```python
from build123d import *

# Parameters (mm, degrees)
F0_R     = 1.6
F1_DEPTH = 3


with BuildPart() as f1:
    # F0 (on Top) → F1 (new body)
    with BuildSketch(Plane.XY):
        with BuildLine():
            ThreePointArc((19.037183, -8.147739), (21.912225, -8.930193), (24.043754, -6.848203))
            ThreePointArc((24.043754, -6.848203), (24.759784, -3.457322), (25, 0))
            ThreePointArc((25, 0), (-19.952507, 15.063116), (6.848203, -24.043754))
            ThreePointArc((6.848203, -24.043754), (8.930193, -21.912225), (8.147739, -19.037183))
            Line((8.147739, -19.037183), (-5.444722, -5.444722))
            ThreePointArc((-5.444722, -5.444722), (-5.444722, 5.444722), (5.444722, 5.444722))
            Line((5.444722, 5.444722), (19.037183, -8.147739))
        make_face()
        with Locations((0, -20)):
            Circle(F0_R, mode=Mode.SUBTRACT)
        with Locations((-20, 0)):
            Circle(F0_R, mode=Mode.SUBTRACT)
        with Locations((20, 0)):
            Circle(F0_R, mode=Mode.SUBTRACT)
        with Locations((0, 20)):
            Circle(F0_R, mode=Mode.SUBTRACT)
        with BuildLine():
            ThreePointArc((6.848203, -24.043754), (17.67767, -17.67767), (24.043754, -6.848203))
            ThreePointArc((24.043754, -6.848203), (21.912225, -8.930193), (19.037183, -8.147739))
            Line((19.037183, -8.147739), (5.444722, 5.444722))
            ThreePointArc((5.444722, 5.444722), (7.113872, 2.946662), (7.7, 0))
            ThreePointArc((7.7, 0), (2.946662, -7.113872), (-5.444722, -5.444722))
            Line((-5.444722, -5.444722), (8.147739, -19.037183))
            ThreePointArc((8.147739, -19.037183), (8.930193, -21.912225), (6.848203, -24.043754))
        make_face()
    extrude(amount=F1_DEPTH)


solid = f1.part
```
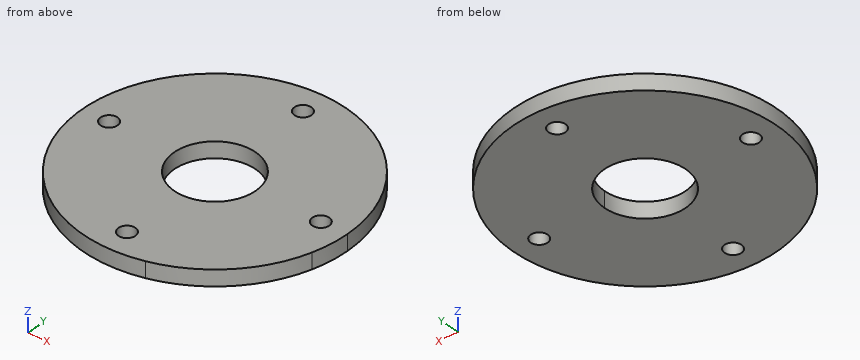
For this review, take the finished solid that the model builds, in its own axes (mm). Coordinates: 2 decimals unless noted, no trailing zeros. Loops run counter-clockwise (first coordinate to the right, second up) from the corner with the lowest first, then second, coordinate; pieces in that order, holes last. Notation, with made-up numbers: (-17.5, -9) - (-11.5, -9) arc R23 cw to (-11.5, -1) - close; hole circle Ø8 at (32.25, 30). An arc over 180 degrees is marked (long way). Use one line per item in the form item = value. Start each with the question number.
1) To check wall thickness, follow probe 1 along Y at (x, z) = (0, 1.3); probe 2 along X at (y, z) = (0.5, 0.2) (3 decimals); probe 3 along Y at (x, z) = (20, 1). State the ranges of each line that lie inside material, in increasing order. Write a range as from..to.
2) Take a section at A-A (y = 20). State the section outline as (x, z) points, plus the area to 3 significant figures.
3) For pin 1 (2.5 mm diameter, centred on x = -20, y = 0, fed in from -Z); pin 2 (4 mm diameter, centred on x = -2.5, y = -17, fed in from -Z); pin 3 (1 mm diameter, centred on x = -8, z = 2, fed in from +Y); pin 4 (1.5 mm diameter, centred on x = 3, z = 2, fed in from -Y), all flat-tipped, find the tip position at first contact; note any pin that passes through.
4) Take a section at B-B (x = 0). State the section outline as (y, z) points, plus the area to 3 significant figures.
5) Take a section at C-C (z = 2.25). State the section outline as (x, y) points.
From the geometry:
q1.probe_1 = -25..-21.6, -18.4..-7.7, 7.7..18.4, 21.6..25
q1.probe_2 = -24.995..-21.52, -18.48..-7.684, 7.684..18.48, 21.52..24.995
q1.probe_3 = -15..-1.6, 1.6..15
q2.outline = (-15, 0) - (-1.6, 0) - (-1.6, 3) - (-15, 3) - close; (1.6, 0) - (15, 0) - (15, 3) - (1.6, 3) - close
q2.area = 80.4 mm2
q3.pin_1 = through
q3.pin_2 = 0
q3.pin_3 = 23.85
q3.pin_4 = -24.9
q4.outline = (-25, 0) - (-21.6, 0) - (-21.6, 3) - (-25, 3) - close; (-18.4, 0) - (-7.7, 0) - (-7.7, 3) - (-18.4, 3) - close; (7.7, 0) - (18.4, 0) - (18.4, 3) - (7.7, 3) - close; (21.6, 0) - (25, 0) - (25, 3) - (21.6, 3) - close
q4.area = 84.6 mm2
q5.outline = (6.85, -24.04) arc R25 ccw to (24.04, -6.85) arc R25 ccw to (25, 0) arc R25 ccw (long way) to start; hole circle Ø3.2 at (-20, 0); hole circle Ø3.2 at (0, -20); hole circle Ø3.2 at (0, 20); hole (5.44, 5.44) arc R7.7 ccw (long way) to (7.7, 0) arc R7.7 ccw to start; hole circle Ø3.2 at (20, 0)
